Part model, mm, in its own coordinate system. A direction names the side the tool comes from. Give positions to 0.01 mm unless a question says otherwise; leave off trailing zeros. Write each loop counter-clockwise with the first axis right and the second up, starting at its lowest first coordinate (ties: lowest second). Pieces come first, ordered by that corner, then holes. Notation, with made-up numbers: M 3,28.5 L 36,28.5 A12 ccw 36,41.5 Z; hole C 17.25,-25 d10. An arc over 180 degrees is marked long. Use a Markdown table: item, result.
```python
from build123d import *

# Parameters (mm, degrees)
BASE_EXTRUSION_DEPTH    = 35
ESQUISSE5_W             = 30
ESQUISSE5_H             = 30
ENL_V_MAT_EXTRU_5_DEPTH = 89.600225733
ESQUISSE6_W             = 25
ESQUISSE6_H             = 20
ENL_V_MAT_EXTRU_6_DEPTH = 99.615414617
ESQUISSE7_R             = 8
ENL_V_MAT_EXTRU_7_DEPTH = 88.177978871


with BuildPart() as part:
    # Esquisse1 → Base-Extrusion (new body)
    with BuildSketch(Plane.XY):
        with BuildLine():
            Line((-60, 0), (-60, -60))
            Line((-60, -60), (-5, -60))
            Line((-5, -60), (-5, 0))
            ThreePointArc((-5, 0), (-32.5, 10), (-60, 0))
        make_face()
    extrude(amount=BASE_EXTRUSION_DEPTH)

    # Esquisse5 → Enlèv. mat.-Extru.5 (cut, through all)
    with BuildSketch(Plane.ZY.offset(60)):
        with Locations((27, -5)):
            Rectangle(ESQUISSE5_W, ESQUISSE5_H)
    extrude(amount=-ENL_V_MAT_EXTRU_5_DEPTH, mode=Mode.SUBTRACT)

    # Esquisse6 → Enlèv. mat.-Extru.6 (cut, through all)
    with BuildSketch(Plane.XZ.offset(60)):
        with Locations((-32.5, 30)):
            Rectangle(ESQUISSE6_W, ESQUISSE6_H)
    extrude(amount=-ENL_V_MAT_EXTRU_6_DEPTH, mode=Mode.SUBTRACT)

    # Esquisse7 → Enlèv. mat.-Extru.7 (cut, through all)
    with BuildSketch(Plane.XY.offset(20)):
        with Locations((-32.5, -43)):
            Circle(ESQUISSE7_R)
    extrude(amount=-ENL_V_MAT_EXTRU_7_DEPTH, mode=Mode.SUBTRACT)


solid = part.part
```
1. Cut at B-B, the plane z = 29. Give the cut face in (x, y), then the cut area to 3 significant figures.
Findings below:
| item | result |
|---|---|
| outline | M -60,-60 L -45,-60 L -45,-20 L -60,-20 Z; M -20,-60 L -5,-60 L -5,-20 L -20,-20 Z |
| area | 1,200 mm2 |
2. Tool access for faces 1 (the flat face through (-53, -40, 35)), 2 (the flat face through (-33, -20, 18)), 3 (the flat face through (-20, -40, 27)): list every direction of +Z, -Z, +X, -X, +Y, -Y with a clear straight run to the whole face (end or side of a thin tool).
Findings below:
| item | result |
|---|---|
| face 1 | +Z, +X, -X, +Y, -Y |
| face 2 | +Z, +X, -X, +Y |
| face 3 | +Z, +Y, -Y |
3. Drill centre lines: L1, parallel to Y at x = -32.5, z = 10.25; L2, parallel to Y at x = -32, z = 13; L3, parallel to X at y = -46.5, z = 22. Where is each one in solid material? Low to high.
Findings below:
| item | result |
|---|---|
| L1 | -60 to -51, -35 to 10 |
| L2 | -60 to -50.98, -35.02 to -20 |
| L3 | -60 to -45, -20 to -5 |
4. Cut at A-A, the plane y = -43. Give the cut face in (x, z), then the cut area to 3 significant figures.
Findings below:
| item | result |
|---|---|
| outline | M -60,0 L -40.5,0 L -40.5,20 L -45,20 L -45,35 L -60,35 Z; M -24.5,0 L -5,0 L -5,35 L -20,35 L -20,20 L -24.5,20 Z |
| area | 1,230 mm2 |
5. Drop flat-ended pins along their axis: P1, Ø3, axis at x = -43, z = 28, coming from the +Y side; P2, Ø24, axis at x = -44, y = -6, coming from the +Z side; P3, Ø12, axis at x = -49, z = 11, coming from the +Y side; P4, Ø8, axis at x = -36, z = 15, coming from the +Y side. Give the stop position or say it passes through.
Findings below:
| item | result |
|---|---|
| P1 | through |
| P2 | z = 12 |
| P3 | y = 8.69 |
| P4 | y = 9.99 |
6. Cut at D-D, the plane y = -32. Give the cut face in (x, z).
Findings below:
| item | result |
|---|---|
| outline | M -60,0 L -5,0 L -5,35 L -20,35 L -20,20 L -45,20 L -45,35 L -60,35 Z |
7. Two-plate mould, pull along Y, no slides. Class faces 4 (the flat face through (-33, -60, 13)), 5 (the flat face through (-45, -40, 27)), 6 (the cylindrical face through (-38.4, -37.6, 10.1)): released by +Y, released by -Y, zero draft, split by the parting line, or undercut.
Findings below:
| item | result |
|---|---|
| face 4 | released by -Y |
| face 5 | zero draft |
| face 6 | undercut |
8. Cut at C-C, the plane x = -32.5. Give the cut face in (y, z), then the cut area to 3 significant figures.
Findings below:
| item | result |
|---|---|
| outline | M -60,0 L -51,0 L -51,20 L -60,20 Z; M -35,0 L 10,0 L 10,12 L -20,12 L -20,20 L -35,20 Z |
| area | 840 mm2 |
